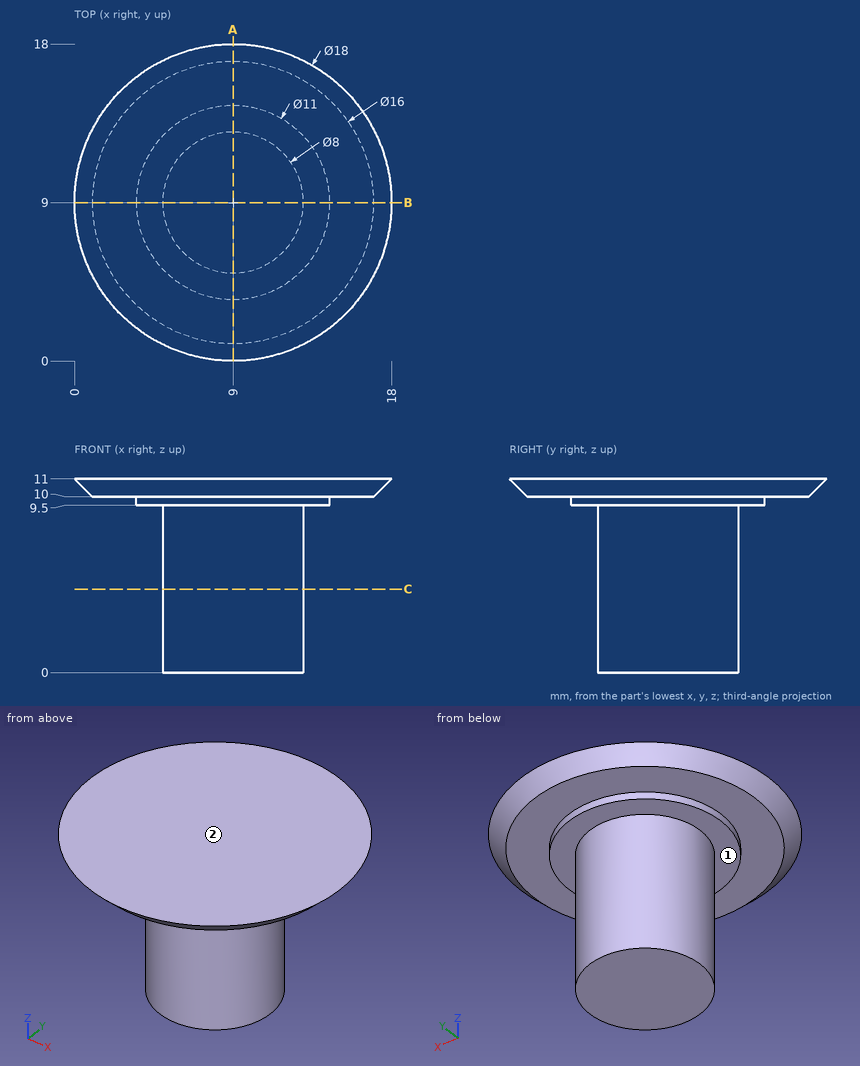
The drawing under review shows one solid part. Ordinate dimensions are in mm from its lowest x, y, z. A direction names the side the tool comes from. Coordinates: 2 decimals unless noted, no trailing zeros. Order: outer loops, then holes, each group sorted by start corner. A loop starts at its lowest first (then second) coordinate and runs counter-clockwise, first axis right, second up. Notation, with made-up numbers: (80, 22.5) -> (114, 22.5) arc R30 cw to (114, 53.5) -> close; hole circle Ø11 at (47, 48.25). An arc over 180 degrees is marked (long way). Answer as CSV lines item,"result".
Q1. We need section C-C (z = 4.75). State the section outline as (x, y) points.
Model answer:
outline,"circle Ø8 at (9, 9)"
Q2. Wall thickness on line 1 along Z through (x, y) = (4.75, 4.5); line 2 along X through (y, z) = (7.5, 5.25); line 3 along Z through (x, y) = (13, 1.75): over which ranges is each line inside the solid? List them lowest first. Write a range as [from, to].
Model answer:
line 1,"z = [10, 11]"
line 2,"x = [5.29, 12.71]"
line 3,"z = [10.28, 11]"
Q3. For the marked faces 1 and 2, list the 3-axis set-ups (+Z, -Z, +X, -X, +Y, -Y) from which the entire face can be reached by the end or side of a thin tool; tool diameter is ignored.
Model answer:
face 1,"-Z"
face 2,"+Z, +X, -X, +Y, -Y"
Q4. We need section A-A (x = 9). State the section outline as (y, z) points, plus the area to 3 significant figures.
Model answer:
outline,"(0, 11) -> (1, 10) -> (3.5, 10) -> (3.5, 9.5) -> (5, 9.5) -> (5, 0) -> (13, 0) -> (13, 9.5) -> (14.5, 9.5) -> (14.5, 10) -> (17, 10) -> (18, 11) -> close"
area,"98.5 mm2"
Q5. Clearance check with flat-ended pins moving along their axes: pin 1 Ø5 at (y, z) = (7.5, 8) entering from +X; pin 2 Ø5 at (x, z) = (2, 2) entering from -Y; pin 3 Ø4 at (y, z) = (3.5, 6.5) entering from -X. State where each tip first meets the part, or that it passes through.
Model answer:
pin 1,"stops at x = 17.4"
pin 2,"passes through"
pin 3,"stops at x = 7.06"
